from build123d import *

# Parameters (mm, degrees)
EXTRUDE_1_DEPTH     = 6.25
CUT_EXTRUDE_1_DEPTH = 12.5
EXTRUDE_2_DEPTH     = 4.24
SKETCH_4_R          = 2.5
SKETCH_4_R_2        = 0.9
EXTRUDE_3_DEPTH     = 3.14
SKETCH_5_R          = 2.5
CUT_EXTRUDE_2_DEPTH = 1
CUT_EXTRUDE_3_REACH = 30.418


with BuildPart() as part:
    # 草图1 → 凸台-拉伸1 (new, symmetric)
    with BuildSketch(Plane(origin=(0, 0, 0), x_dir=(0, 0, -1), z_dir=(1, 0, 0))):
        Polygon((-11.3, 4.28), (11.3, 4.28), (11.3, 0), (16.2, 0), (16.2, -2.46), (11.3, -2.46), (11.3, -19.72), (-11.3, -19.72), (-11.3, -2.46), (-16.2, -2.46), (-16.2, 0), (-11.3, 0), align=None)
    extrude(amount=EXTRUDE_1_DEPTH, both=True)

    # 草图2 → 切除-拉伸1 (cut)
    with BuildSketch(Plane(origin=(0, 0, 0), x_dir=(1, 0, 0), z_dir=(0, 1, 0))):
        with BuildLine():
            Line((-0.5, 15), (-0.5, 16.2))
            Line((-0.5, 16.2), (0.5, 16.2))
            Line((0.5, 16.2), (0.5, 15))
            ThreePointArc((0.5, 15), (0, 12.5), (-0.5, 15))
        make_face()
        with BuildLine():
            Line((-0.5, -15), (-0.5, -16.2))
            Line((-0.5, -16.2), (0.5, -16.2))
            Line((0.5, -16.2), (0.5, -15))
            ThreePointArc((0.5, -15), (0, -12.5), (-0.5, -15))
        make_face()
    extrude(amount=-CUT_EXTRUDE_1_DEPTH, mode=Mode.SUBTRACT)

    # 草图3 → 凸台-拉伸2 (add)
    with BuildSketch(Plane(origin=(0, 4.28, 0), x_dir=(1, 0, 0), z_dir=(0, 1, 0))):
        with BuildLine():
            ThreePointArc((2.794246193, -0.540589255), (0, 11.3), (-2.794246193, -0.540589255))
            ThreePointArc((-2.794246193, -0.540589255), (0, -3.52), (2.794246193, -0.540589255))
        make_face()
    extrude(amount=EXTRUDE_2_DEPTH)

    # 草图4 → 凸台-拉伸3 (add)
    with BuildSketch(Plane(origin=(0, 8.52, 0), x_dir=(1, 0, 0), z_dir=(0, 1, 0))):
        with Locations(Location((0, 5.05, 0), (0, 0, 270))):
            Circle(SKETCH_4_R)
        with Locations(Location((0, 5.05, 0), (0, 0, 270))):
            Circle(SKETCH_4_R_2, mode=Mode.SUBTRACT)
    extrude(amount=EXTRUDE_3_DEPTH)

    # 草图5 → 切除-拉伸2 (cut)
    with BuildSketch(Plane.XZ.offset(19.72)):
        with Locations((6.25, 11.3)):
            Circle(SKETCH_5_R)
        with Locations((6.25, -11.3)):
            Circle(SKETCH_5_R)
        with Locations((-6.25, -11.3)):
            Circle(SKETCH_5_R)
        with Locations((-6.25, 11.3)):
            Circle(SKETCH_5_R)
    extrude(amount=-CUT_EXTRUDE_2_DEPTH, mode=Mode.SUBTRACT)

    # 切除-拉伸3: up to this face of the body (flat: up to its plane)
    cut_extrude_3_end = Plane(part.part.faces().sort_by_distance((6.25, -7.338953034, 0))[0])
    # 草图6 → 切除-拉伸3 (cut, up to the picked face)
    with BuildSketch(Plane.ZY.offset(6.25), mode=Mode.PRIVATE) as cut_extrude_3_sk1:
        Polygon((-11.3, -18.72), (-11.3, -19.72), (-8.3, -19.72), align=None)
    cut_extrude_3_tool1 = split(extrude(cut_extrude_3_sk1.sketch, amount=-CUT_EXTRUDE_3_REACH, mode=Mode.PRIVATE), bisect_by=cut_extrude_3_end, keep=Keep.BOTH, mode=Mode.PRIVATE)
    add(cut_extrude_3_tool1.solids().sort_by(Axis((-6.25, -19.386667, -10.3), (1, 0, 0)))[0], mode=Mode.SUBTRACT)


solid = part.part
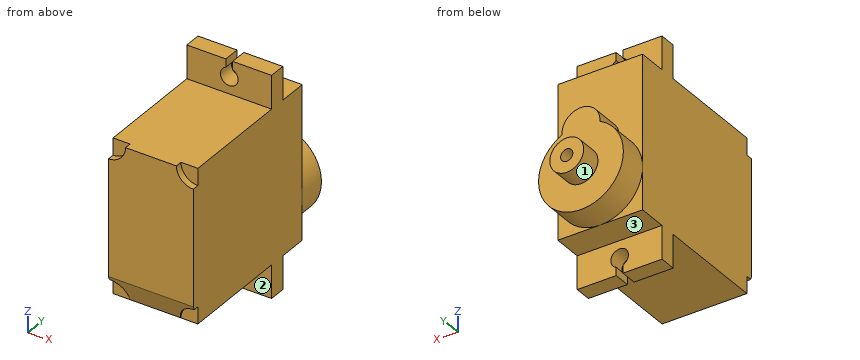
Geometry check sheet. Reference: the model listing, model coordinates, mm. Face numbers are marked on the shaded views. A direction names the side the tool comes from. Round coordinates to 2 decimals unless told otherwise and drop trailing zeros. Loops run counter-clockwise (first coordinate to the right, second up) from the corner with the lowest first, then second, coordinate; pieces in that order, holes last.
Item 1: Cross-section at C-C on y = 9. Record the boundary of the cut face in (x, z).
Item 2: Cross-section at D-D on z = -12. Record the boundary of the cut face in (x, y).
Item 3: Access from +Z, -Z, +X, -X, +Y, -Y to the whole of each face (thin tool, end or side, straight path). Record for the marked faces 1, 2 and 3.
Item 4: Cross-section at B-B on x = -3.25. Record the boundary of the cut face in (y, z).
Item 5: Gauge pin test, flat ends, axial feed: pin 1 (5 mm diameter, centred on x = -1, z = 7.5, fed in from +Y); pin 2 (2.5 mm diameter, centred on x = -1, z = 14.5, fed in from -Y); pin 3 (2 mm diameter, centred on x = -1, y = 4, fed in from -Z). Record the tip position at first contact, or that the pin passes through.
Item 6: Thickness scan on line 1 (X direction, y = -1.05, z = -13.8); line 2 (X direction, y = 10.75, z = -5.05); line 3 (Y direction, x = 5, z = 8). Record the ranges inside material, lowest first.
Item 7: Cross-section at A-A on z = 13.8. Record the boundary of the cut face in (x, y).
Answer sheet:
1. outline: circle Ø5 at (0, -5.05); hole circle Ø1.8 at (0, -5.05)
2. outline: (-6.25, -2.46) - (6.25, -2.46) - (6.25, 0) - (-6.25, 0) - close
3. face 1: +Y
3. face 2: -Z, +X, -X, -Y
3. face 3: -Z, +X, -X, +Y
4. outline: (-19.72, -8.3) - (-18.72, -11.3) - (-2.46, -11.3) - (-2.46, -16.2) - (0, -16.2) - (0, -11.3) - (4.28, -11.3) - (4.28, -10.39) - (8.52, -10.39) - (8.52, 0.29) - (4.28, 0.29) - (4.28, 11.3) - (0, 11.3) - (0, 16.2) - (-2.46, 16.2) - (-2.46, 11.3) - (-19.72, 11.3) - close
5. pin 1: stops at y = 4.28
5. pin 2: stops at y = -2.46
5. pin 3: stops at z = -11.3
6. line 1: x = -6.25 to -1.3, 1.3 to 6.25
6. line 2: x = -2.5 to -0.9, 0.9 to 2.5
6. line 3: y = -19.72 to 4.28
7. outline: (-6.25, -2.46) - (-1.3, -2.46) - (-1.3, 0) - (-6.25, 0) - close; (1.3, -2.46) - (6.25, -2.46) - (6.25, 0) - (1.3, 0) - close
